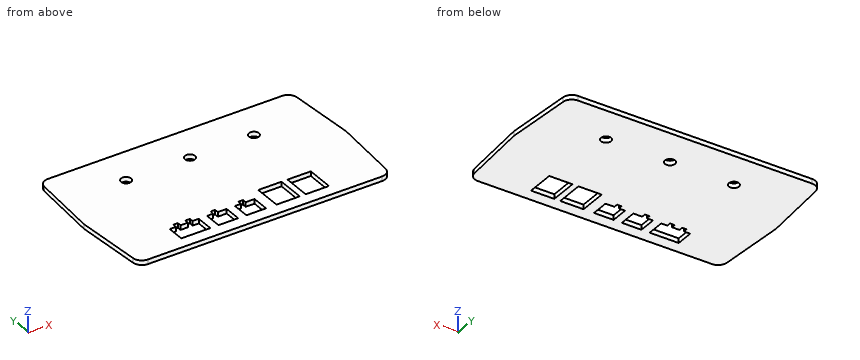
```python
from build123d import *

# Parameters (mm, degrees)
F0_W     = 12.75
F0_H     = 15
F0_R     = 2.75
F1_DEPTH = 2.5
F2_R     = 1.5


with BuildPart() as f1:
    # F0 (on Top) → F1 (new body)
    with BuildSketch(Plane.XY):
        with BuildLine():
            ThreePointArc((69.087259747, 36.6126784789), (67.5053247579, 39.9115155602), (64.1004306622, 41.25))
            Line((64.1004306622, 41.25), (-64.1004306622, 41.25))
            ThreePointArc((-64.1004306622, 41.25), (-67.5053247579, 39.9115155602), (-69.087259747, 36.6126784789))
            Line((-69.087259747, 36.6126784789), (-71.75, 0))
            Line((-71.75, 0), (-69.087259747, -36.6126784789))
            ThreePointArc((-69.087259747, -36.6126784789), (-67.5053247579, -39.9115155602), (-64.1004306622, -41.25))
            Line((-64.1004306622, -41.25), (64.1004306622, -41.25))
            ThreePointArc((64.1004306622, -41.25), (67.5053247579, -39.9115155602), (69.087259747, -36.6126784789))
            Line((69.087259747, -36.6126784789), (71.75, 0))
            Line((71.75, 0), (69.087259747, 36.6126784789))
        make_face()
        Polygon((-25.55, -25.15), (-25.55, -34.65), (-41.45, -34.65), (-41.45, -25.15), (-38.05, -25.15), (-38.05, -22.95), (-35.55, -22.95), (-35.55, -25.15), (-31.45, -25.15), (-31.45, -22.95), (-28.95, -22.95), (-28.95, -25.15), align=None, mode=Mode.SUBTRACT)
        Polygon((-10.3, -25.15), (-10.3, -34.65), (-21.05, -34.65), (-21.05, -25.15), (-17.65, -25.15), (-17.65, -22.95), (-15.15, -22.95), (-15.15, -25.15), align=None, mode=Mode.SUBTRACT)
        Polygon((4.95, -25.15), (4.95, -34.65), (-5.8, -34.65), (-5.8, -25.15), (-2.4, -25.15), (-2.4, -22.95), (0.1, -22.95), (0.1, -25.15), align=None, mode=Mode.SUBTRACT)
        with Locations((17.025, -27.15)):
            Rectangle(F0_W, F0_H, mode=Mode.SUBTRACT)
        with Locations((33.025, -27.15)):
            Rectangle(F0_W, F0_H, mode=Mode.SUBTRACT)
        with Locations((-35, 20.625)):
            Circle(F0_R, mode=Mode.SUBTRACT)
        with Locations((0, 20.625)):
            Circle(F0_R, mode=Mode.SUBTRACT)
        with Locations((35, 20.625)):
            Circle(F0_R, mode=Mode.SUBTRACT)
    extrude(amount=F1_DEPTH)

    # F2
    f2_edges = [f1.edges().sort_by_distance(p)[0] for p in [
        (-71.75, 0, 1.25),
        (71.75, 0, 1.25),
    ]]
    fillet(f2_edges, radius=F2_R)


solid = f1.part
```
Part model, mm, in its own coordinate system. Round coordinates to 2 decimals unless told otherwise and drop trailing zeros. Write each loop counter-clockwise with the first axis right and the second up, starting at its lowest first coordinate (ties: lowest second). Pieces come first, ordered by that corner, then holes.
Item 1: Drop flat-ended pins along their axis: pin 1 Ø1.2 at (y, z) = (-29.5, 0.5) entering from -X; pin 2 Ø0.7 at (y, z) = (-24.5, 1.5) entering from +X; pin 3 Ø1.1 at (y, z) = (-24, 1) entering from -X. Give the stop position or say it passes through.
Results:
pin 1: stops at x = -69.65
pin 2: stops at x = 69.99
pin 3: stops at x = -70.04
Item 2: Cut at B-B, the plane x = -34. Give the cut face in (y, z).
Results:
outline: (-41.25, 0) - (-34.65, 0) - (-34.65, 2.5) - (-41.25, 2.5) - close; (-25.15, 0) - (18.06, 0) - (18.06, 2.5) - (-25.15, 2.5) - close; (23.19, 0) - (41.25, 0) - (41.25, 2.5) - (23.19, 2.5) - close
Item 3: Cut at C-C, the plane z = 1.6. Count the separate pieces of the cut face and the enclosed holes in it, plus the area to 3 significant figures.
Results:
separate pieces: 1
enclosed holes: 8
area: 10,700 mm2
Item 4: Probe L1, parallel to Y at x = 35, z = 0.95 (3 decimals); L2, parallel to Y at x = -16, z = 0.6; L3, parallel to Y at x = -35, z = 1.9 (3 decimals). List the from-to ranges inside material, lowest first.
Results:
L1: y = -41.25 to -34.65, -19.65 to 17.875, 23.375 to 41.25
L2: y = -41.25 to -34.65, -22.95 to 41.25
L3: y = -41.25 to -34.65, -25.15 to 17.875, 23.375 to 41.25
Item 5: Cut at A-A, the plane x = 35. Give the cut face in (y, z) (3 decimals).
Results:
outline: (-41.25, 0) - (-34.65, 0) - (-34.65, 2.5) - (-41.25, 2.5) - close; (-19.65, 0) - (17.875, 0) - (17.875, 2.5) - (-19.65, 2.5) - close; (23.375, 0) - (41.25, 0) - (41.25, 2.5) - (23.375, 2.5) - close
